Job drawing, mm, ordinate dimensions from the low corner. One solid piece. A direction names the side the tool comes from. Coordinates: 2 decimals unless noted, no trailing zeros. Write each loop counter-clockwise with the first axis right and the second up, starting at its lowest first coordinate (ties: lowest second). Pieces come first, ordered by that corner, then holes. Notation, with made-up numbers: (39.5, 68) - (69.5, 68) arc R26 cw to (69.5, 91) - close; hole circle Ø10 at (84, 56). An arc over 180 degrees is marked (long way). Use a Markdown table: item, result.
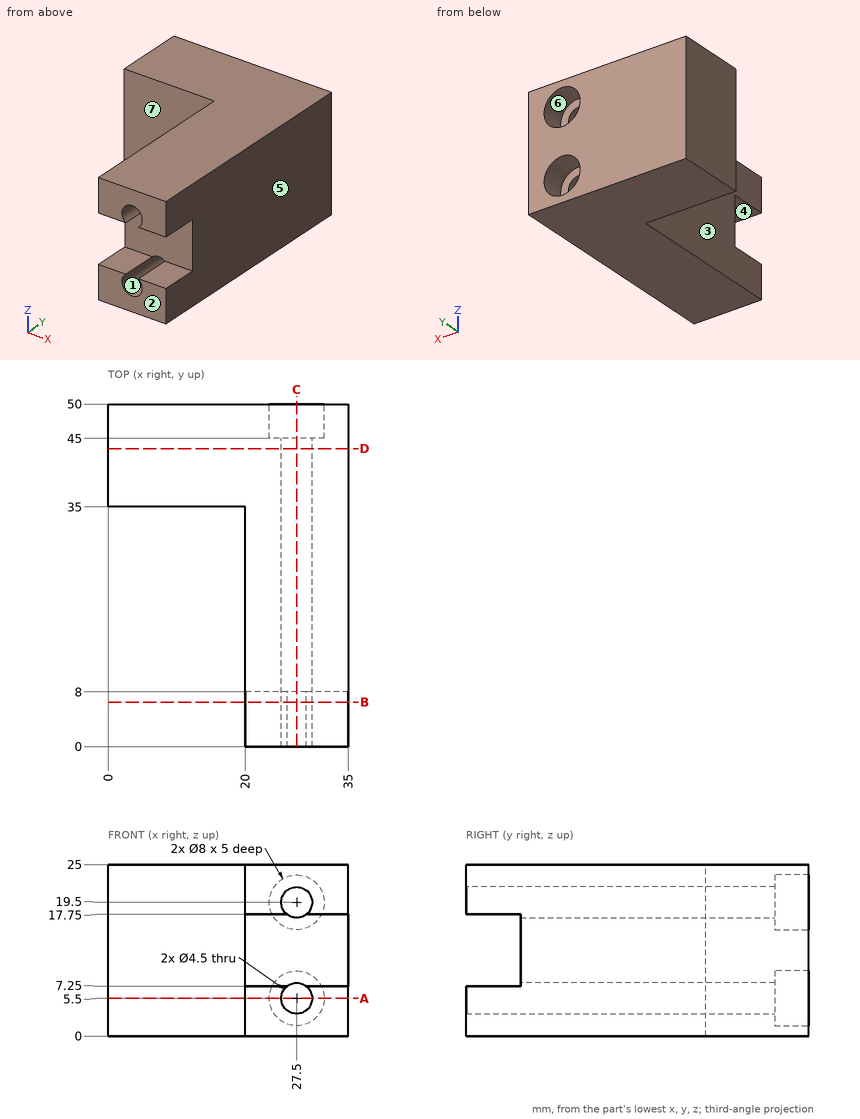
Item 1: Drill centre lines: probe 1 along Z at (x, y) = (27.5, 12.5); probe 2 along X at (y, z) = (29, 19.5); probe 3 along X at (y, z) = (47.7, 5.5). Where is each one in solid material? Low to high.
From the geometry:
| item | result |
|---|---|
| probe 1 | 0 to 3.25, 7.75 to 17.25, 21.75 to 25 |
| probe 2 | 20 to 25.25, 29.75 to 35 |
| probe 3 | 0 to 23.5, 31.5 to 35 |
Item 2: Band-saw the part on D-D, the plane y = 43.5. Give the cut face in (x, z), then the cut area to 3 significant figures.
From the geometry:
| item | result |
|---|---|
| outline | (0, 0) - (35, 0) - (35, 25) - (0, 25) - close; hole circle Ø4.5 at (27.5, 5.5); hole circle Ø4.5 at (27.5, 19.5) |
| area | 843 mm^2 |
Item 3: Band-saw the part on C-C, the plane x = 27.5. Give the cut face in (y, z).
From the geometry:
| item | result |
|---|---|
| outline | (0, 0) - (50, 0) - (50, 1.5) - (45, 1.5) - (45, 3.25) - (0, 3.25) - close; (0, 21.75) - (45, 21.75) - (45, 23.5) - (50, 23.5) - (50, 25) - (0, 25) - close; (8, 7.75) - (45, 7.75) - (45, 9.5) - (50, 9.5) - (50, 15.5) - (45, 15.5) - (45, 17.25) - (8, 17.25) - close |
Item 4: Band-saw the part on A-A, the plane z = 5.5. Give the cut face in (x, y).
From the geometry:
| item | result |
|---|---|
| outline | (0, 35) - (20, 35) - (20, 0) - (25.25, 0) - (25.25, 45) - (23.5, 45) - (23.5, 50) - (0, 50) - close; (29.75, 0) - (35, 0) - (35, 50) - (31.5, 50) - (31.5, 45) - (29.75, 45) - close |
Item 5: Two-plate mould, pull along X, no slides. Class the marked faces 1, 2 and 3: pulls with the +X half, pulls with the -X half, needs draft (parallel to the pull), parting line crosses it, or undercut.
From the geometry:
| item | result |
|---|---|
| face 1 | undercut |
| face 2 | needs draft |
| face 3 | pulls with the -X half |
Item 6: Band-saw the part on B-B, the plane y = 6.5. Give the cut face in (x, z).
From the geometry:
| item | result |
|---|---|
| outline | (20, 0) - (35, 0) - (35, 7.25) - (28.91, 7.25) arc R2.25 cw (long way) to (26.09, 7.25) - (20, 7.25) - close; (20, 17.75) - (26.09, 17.75) arc R2.25 cw (long way) to (28.91, 17.75) - (35, 17.75) - (35, 25) - (20, 25) - close |
Item 7: Which spindle directions (+Z, -Z, +X, -X, +Y, -Y) get a long thin tool onto all of the face, cutting with end or side? Do the marked faces 4, 5, 6 and 7. Say none if no direction does.
From the geometry:
| item | result |
|---|---|
| face 4 | +X, -X, -Y |
| face 5 | +Z, -Z, +X, +Y, -Y |
| face 6 | +Y |
| face 7 | +Z, -Z, -X, -Y |
Item 8: Drop flat-ended pins along their axis: P1, Ø5, axis at y = 30.5, z = 10, coming from the -X side; P2, Ø10, axis at x = 14.5, z = 12, coming from the -Y side. Give the stop position or say it passes through.
From the geometry:
| item | result |
|---|---|
| P1 | x = 20 |
| P2 | y = 35 |
